The model under review builds one solid part; all positions refer to its coordinate system, in mm. Round coordinates to 2 decimals unless told otherwise and drop trailing zeros. Loops run counter-clockwise (first coordinate to the right, second up) from the corner with the lowest first, then second, coordinate; pieces in that order, holes last. Notation, with made-up numbers: M 83.5,53 L 116.5,53 A19 cw 116.5,72 Z; hole C 72,51 d4. An arc over 180 degrees is marked long. Answer as a JSON object with one key per item and string values. Group by question number.
Item 1: Consider section C-C (z = 58.5). Give the boundary of the cut face in (x, y), and give its area (3 significant figures).
Item 2: Consider section D-D (y = -4.25). Give the boundary of the cut face in (x, z).
Item 3: To check wall thickness, follow line 1 (Z direction, x = -0.5, y = 2.5); line 2 (X direction, y = 5.75, z = 8.5); line 3 (X direction, y = 2.75, z = 2.5). State the ranges of each line that lie inside material, in increasing order.
Item 4: Consider section A-A (y = 2.5). Give the boundary of the cut face in (x, z), and give its area (3 significant figures).
Item 5: Consider section B-B (x = 0). Give the boundary of the cut face in (y, z), and give its area (3 significant figures).
Item 6: Insertion check: P1, Ø4, axis at y = 2.5, z = 33, coming from the +X side; P2, Ø1.8, axis at y = 3.5, z = 5, coming from the -X side; P3, Ø1.5, axis at x = -3, z = 31.5, coming from the -Y side. Each pin has a flat end and moves straight along its axis. Give the tip position at first contact, or say it passes through.
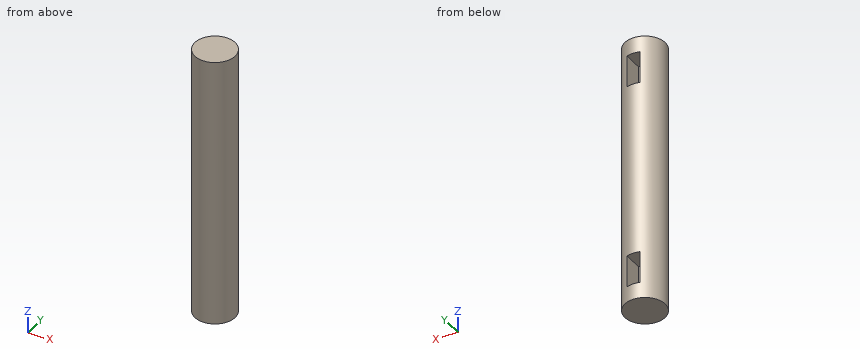
```python
from build123d import *

# Parameters (mm, degrees)
BOSS_EXTRUDE1_DEPTH      = 80
BOSS_EXTRUDE1_DEPTH_BACK = 5
SKETCH1_R                = 6.3
CUT_EXTRUDE1_DEPTH       = 10


with BuildPart() as part:
    # Sketch1 → Boss-Extrude1 (new, two sides: drawn at the far end of the back side and taken through both)
    with BuildSketch(Plane.XY.offset(-BOSS_EXTRUDE1_DEPTH_BACK)):
        Circle(SKETCH1_R)
    extrude(amount=BOSS_EXTRUDE1_DEPTH + BOSS_EXTRUDE1_DEPTH_BACK)

    # Sketch6 → Cut-Extrude1 (cut)
    with BuildSketch(Plane(origin=(0, 0, 0), x_dir=(1, 0, 0), z_dir=(0, 1, 0))):
        Polygon((-1.955160092, -70), (-1.955160092, -65.008101893), (0, -65.008101893), (2.038358394, -65.008101893), (2.038358394, -74.991898107), (-1.955160092, -74.991898107), align=None)
        Polygon((0, 0), (-1.955160092, 0), (-1.955160092, -10), (2.038358394, -10), (2.038358394, 0), align=None)
    extrude(amount=CUT_EXTRUDE1_DEPTH, mode=Mode.SUBTRACT)


solid = part.part
```
Geometry results:
{
 "1": {"outline": "C 0,0 d12.6", "area": "125 mm^2"},
 "2": {"outline": "M -4.65,-5 L 4.65,-5 L 4.65,80 L -4.65,80 Z"},
 "3": {"line 1": "z = -5 to 0, 10 to 65.01, 74.99 to 80", "line 2": "x = -2.57 to -1.96, 2.04 to 2.57", "line 3": "x = -5.67 to -1.96, 2.04 to 5.67"},
 "4": {"outline": "M -5.78,-5 L 5.78,-5 L 5.78,80 L -5.78,80 Z; hole M -1.96,0 L 2.04,0 L 2.04,10 L -1.96,10 Z; hole M -1.96,65.01 L 2.04,65.01 L 2.04,74.99 L -1.96,74.99 Z", "area": "903 mm^2"},
 "5": {"outline": "M -6.3,-5 L 6.3,-5 L 6.3,0 L 0,0 L 0,10 L 6.3,10 L 6.3,65.01 L 0,65.01 L 0,74.99 L 6.3,74.99 L 6.3,80 L -6.3,80 Z", "area": "945 mm^2"},
 "6": {"P1": "stops at x = 6.28", "P2": "stops at x = -5.74", "P3": "stops at y = -5.88"}
}
